```python
from build123d import *

# Parameters (mm, degrees)
F0_W     = 508
F0_H     = 508
F0_R     = 190.5
F1_DEPTH = 15
F2_SIZE  = 5.08


with BuildPart() as f1:
    # F0 (on Top) → F1 (new body)
    with BuildSketch(Plane.XY):
        Rectangle(F0_W, F0_H)
        Circle(F0_R, mode=Mode.SUBTRACT)
    extrude(amount=F1_DEPTH)

    # F2
    f2_edges = [f1.edges().sort_by_distance(p)[0] for p in [
        (-190.5, 0, 15),
    ]]
    chamfer(f2_edges, length=F2_SIZE)


solid = f1.part
```
Input: part model. Units: mm. Frame: model coordinates. Coordinates: 2 decimals unless noted, no trailing zeros. Loops run counter-clockwise (first coordinate to the right, second up) from the corner with the lowest first, then second, coordinate; pieces in that order, holes last. Notation, with made-up numbers: M -9.75,-4 L -5.75,-4 A30 cw -5.75,34 Z; hole C 56,80.25 d11. An arc over 180 degrees is marked long. Answer in a Markdown table with one row per item.
1. Material intervals for line 1 (Y direction, x = 0, z = 6); line 2 (Y direction, x = 61.5, z = 10.5); line 3 (X direction, y = -120, z = 5), sorted ascending.
Response:
| item | result |
|---|---|
| line 1 | y = -254 to -190.5, 190.5 to 254 |
| line 2 | y = -254 to -180.91, 180.91 to 254 |
| line 3 | x = -254 to -147.95, 147.95 to 254 |
2. Section A-A, the plane y = 0. Output: boundary loops of the cut face in (x, z), then the cut area to 3 significant figures.
Response:
| item | result |
|---|---|
| outline | M -254,0 L -190.5,0 L -190.5,9.92 L -195.58,15 L -254,15 Z; M 190.5,0 L 254,0 L 254,15 L 195.58,15 L 190.5,9.92 Z |
| area | 1,880 mm2 |
3. Draft query along X for faces 1 (the cylindrical face through (-151.17, -115.92, 4.89)), 2 (the conical face through (182.01, 57.32, 10.24)), 3 (the flat face through (-4, 254, 7)), 4 (the flat face through (-254, -4, 7)). Return one class per face: pulls with the +X half, pulls with the -X half, needs draft (parallel to the pull), parting line crosses it, or undercut.
Response:
| item | result |
|---|---|
| face 1 | undercut |
| face 2 | undercut |
| face 3 | needs draft |
| face 4 | pulls with the -X half |
